```python
from build123d import *

# Parameters (mm, degrees)
F1_DEPTH = 52
F3_DEPTH = 20
F4_R     = 10
F5_DEPTH = 25


with BuildPart() as f1:
    # F0 (on Front) → F1 (new body)
    with BuildSketch(Plane.XZ):
        Polygon((0, 0), (-64.8528137424, 64.8528137424), (-78.9949493661, 50.7106781187), (-8.2842712475, -20), (111.7157287525, -20), (111.7157287525, 0), align=None)
    extrude(amount=F1_DEPTH)

    # F2 (on face) → F3 (cut, through all)
    with BuildSketch(Plane.XY):
        with BuildLine():
            Line((21.7918254922, -35.9997104601), (91.7156873447, -36))
            ThreePointArc((91.7156873447, -36), (101.7157283101, -25.9970253962), (91.7097381372, -16.0000017944))
            Line((91.7097381372, -16.0000017944), (22.6246005983, -16.0413880501))
            ThreePointArc((22.6246005983, -16.0413880501), (11.724422575, -25.5831056894), (21.7918254922, -35.9997104601))
        make_face()
    extrude(amount=-F3_DEPTH, mode=Mode.SUBTRACT)

    # F4 (on face) → F5 (cut)
    with BuildSketch(Plane(origin=(0, 0, 0), x_dir=(0.7071067812, 0, -0.7071067812), z_dir=(0.7071067812, 0, 0.7071067812))):
        with BuildLine():
            ThreePointArc((-65.7157287525, -52), (-84.1005050634, -44.3847763109), (-91.7157287525, -26))
            Line((-91.7157287525, -26), (-91.7157287525, -52))
            Line((-91.7157287525, -52), (-65.7157287525, -52))
        make_face()
        with Locations((-65.7157287525, -26)):
            Circle(F4_R)
        with BuildLine():
            ThreePointArc((-91.7157287525, -26), (-84.1005050634, -7.6152236891), (-65.7157287525, 0))
            Line((-65.7157287525, 0), (-91.7157287525, 0))
            Line((-91.7157287525, 0), (-91.7157287525, -26))
        make_face()
    extrude(amount=-F5_DEPTH, mode=Mode.SUBTRACT)


solid = f1.part
```
Geometry check sheet. Reference: the model listing, model coordinates, mm. A direction names the side the tool comes from. Coordinates: 2 decimals unless noted, no trailing zeros. Order: outer loops, then holes, each group sorted by start corner. A loop starts at its lowest first (then second) coordinate and runs counter-clockwise, first axis right, second up.
Q1. Draft check along Y on faces 4 (the face through (11.736, -25.357, -9.86)), 5 (the face through (-32, -26, 32)), 6 (the face through (19, 0, -4)). Enter one of: released by +Y, released by -Y, zero draft, split by the parting line, or undercut.
Reply:
face 4: undercut
face 5: zero draft
face 6: released by +Y
Q2. Depth check by flat-ended pin: pin 1 Ø4 at (y, z) = (-31.5, -5.5) entering from -X; pin 2 Ø1.5 at (x, z) = (-55.5, 50.5) entering from -Y. Enter the tip coordinate at first touch or a pass-through.
Reply:
pin 1: stops at x = -24.78
pin 2: stops at y = -50.58
Q3. Tool access check on faces 1 (the face through (111.716, -26, -10)), 2 (the face through (57, -14, 0)), 3 (the face through (101.713, -26.217, -9.86)). Record the directions out of +Z, -Z, +X, -X, +Y, -Y that give a thin tool (end or side, any length) a straight path to the whole face; none if there is none.
Reply:
face 1: +Z, -Z, +X, +Y, -Y
face 2: +Z, +X, +Y, -Y
face 3: +Z, -Z
Q4. Thickness scan on probe 1 along Y at (x, z) = (39.5, -7); probe 2 along Z at (x, y) = (17, -8); probe 3 along Z at (x, y) = (-35, -18.5). Record the ranges inside material, lowest first.
Reply:
probe 1: y = -52 to -36, -16.03 to 0
probe 2: z = -20 to 0
probe 3: z = 6.72 to 35
Q5. Sectioned sample at C-C on x = 68. Record the cut outline in (y, z), and give its area (3 significant figures).
Reply:
outline: (-52, -20) - (-36, -20) - (-36, 0) - (-52, 0) - close; (-16.01, -20) - (0, -20) - (0, 0) - (-16.01, 0) - close
area: 640 mm2
Q6. Sectioned sample at D-D on y = -9. Record the cut outline in (x, z).
Reply:
outline: (-74.52, 46.24) - (-8.28, -20) - (111.72, -20) - (111.72, 0) - (0, 0) - (-60.38, 60.38) - close
Q7. Sectioned sample at A-A on y = -21. Record the cut outline in (x, z), and give its area (3 significant figures).
Reply:
outline: (-78.65, 50.37) - (-66.73, 38.45) - (-52.59, 52.59) - (-64.51, 64.51) - close; (-54.49, 26.2) - (-8.28, -20) - (13.06, -20) - (13.06, 0) - (0, 0) - (-40.34, 40.34) - close; (100.38, -20) - (111.72, -20) - (111.72, 0) - (100.38, 0) - close
area: 2,130 mm2
Q8. Sectioned sample at B-B on z = -5. Record the cut outline in (x, y).
Reply:
outline: (-23.28, -52) - (111.72, -52) - (111.72, 0) - (-23.28, 0) - close; hole (21.79, -36) - (91.72, -36) arc R10 ccw to (91.71, -16) - (22.62, -16.04) arc R10 ccw (long way) to start
